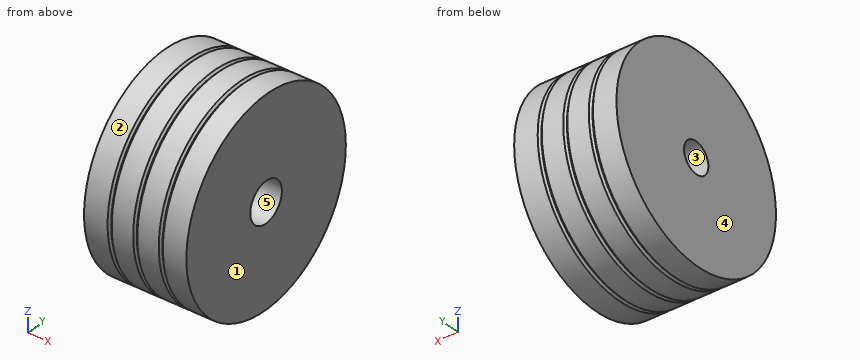
Autodesk Inventor part; units mm, degrees
ref_plane "YZ Plane" through (0, 0, 0) normal (1, 0, 0) x (0, 1, 0)
ref_plane "XZ Plane" through (0, 0, 0) normal (0, 1, 0) x (-1, 0, 0)
ref_plane "XY Plane" through (0, 0, 0) normal (0, 0, 1) x (1, 0, 0)
sketch "Boceto1" plane through (0, 0, 0) normal (0, 0, 1) x (1, 0, 0)
  line L0 (0, 0) -> (-6.35, 0)
  line L1 (-6.35, 0) -> (-6.35, 6.35)
  line L2 (0, 6.35) -> (0, 0)
  line L3 (-4.7625, 6.223) -> (-4.6355, 6.35)
  line L4 (-4.7625, 6.223) -> (-4.5829, 6.223) construction
  line L5 (-4.7625, 6.223) -> (-4.8895, 6.35)
  line L6 (-4.7625, 6.223) -> (-4.5829, 6.223) construction
  line L7 (-3.175, 6.223) -> (-3.048, 6.35)
  line L8 (-3.175, 6.223) -> (-2.9954, 6.223) construction
  line L9 (-3.175, 6.223) -> (-3.302, 6.35)
  line L10 (-3.175, 6.223) -> (-2.9954, 6.223) construction
  line L11 (-1.5875, 6.223) -> (-1.4605, 6.35)
  line L12 (-1.5875, 6.223) -> (-1.4079, 6.223) construction
  line L13 (-1.5875, 6.223) -> (-1.7145, 6.35)
  line L14 (-1.5875, 6.223) -> (-1.4079, 6.223) construction
  line L15 (-6.35, 6.35) -> (-4.8895, 6.35)
  line L16 (-4.6355, 6.35) -> (-3.302, 6.35)
  line L17 (-3.048, 6.35) -> (-1.7145, 6.35)
  line L18 (-1.4605, 6.35) -> (0, 6.35)
  dimension "d0" = 6.35
  dimension "d1" = 6.35
  dimension "d3" = 1.5875
  dimension "d6" = 1.5875
  dimension "d7" = 1.5875
  dimension "d20" = 0.127
revolve "Revolución1" add sketch "Boceto1" angle 360 about axis through (0, 0, 0) along (-1, 0, 0)
sketch "Boceto2" plane through (0, 0, 0) normal (1, 0, 0) x (0, 0, -1)
  point P0 (0, 0)
  point P1 (0, 0)
hole "Agujero1" at (0, 0, 0) direction (-1, 0, 0) diameter 1.9406 end through all counterbore diameter 2.5146 counterbore depth 3.175
equation "\"d7\" = d6"
properties part number "Piston" material "Latón, amarillo claro"
Part model, mm, in its own coordinate system. Face numbers are marked on the shaded views. A direction names the side the tool comes from. Coordinates: 2 decimals unless noted, no trailing zeros. Loops run counter-clockwise (first coordinate to the right, second up) from the corner with the lowest first, then second, coordinate; pieces in that order, holes last. Notation, with made-up numbers: M 20.25,53.5 L 75.25,53.5 A13 ccw 75.25,78.5 Z; hole C 65.25,13 d7. An arc over 180 degrees is marked long. Use a Markdown table: item, result. Add a question column.
Q1. Cut at C-C (x = -5.5). Write the cut outline in (y, z).
Q2. Mould opens along Y. For the marked faces 1, 2 and 3 say: +Y half, -Y half, draft (parallel to the pull), parting line (faces both ways), or undercut.
Q3. Probe L1, parallel to Z at x = -4, y = 0; L2, parallel to Y at x = -1.2, z = 0. List the from-to ranges inside material, lowest first.
Q4. Which spindle directions (+Z, -Z, +X, -X, +Y, -Y) get a long thin tool onto all of the face, cutting with end or side? Do the marked faces 4 and 5. Say none if no direction does.
Q5. Cut at D-D (x = -2). Write the cut outline in (y, z).
Q6. Pin check, flat tips, straight feed: P1, Ø1.5, axis at x = -1.5, z = 2.5, coming from the +Y side; P2, Ø3, axis at x = -4.5, y = 3, coming from the +Z side. Stop position of each tip, or through.
Worked out:
| question | item | result |
|---|---|---|
| 1 | outline | C 0,0 d12.7; hole C 0,0 d1.94 |
| 2 | face 1 | draft |
| 2 | face 2 | parting line |
| 2 | face 3 | undercut |
| 3 | L1 | z = -6.35 to -0.97, 0.97 to 6.35 |
| 3 | L2 | y = -6.35 to -1.26, 1.26 to 6.35 |
| 4 | face 4 | +Z, -Z, -X, +Y, -Y |
| 4 | face 5 | +X |
| 5 | outline | C 0,0 d12.7; hole C 0,0 d2.51 |
| 6 | P1 | stops at y = 6.1 |
| 6 | P2 | stops at z = 6.17 |
